Read the model definition and answer for the solid it produces. Units are mm, in the model's axes. A direction names the side the tool comes from. Round coordinates to 2 decimals unless told otherwise and drop trailing zeros. Order: outer loops, then holes, each group sorted by start corner. A loop starts at its lowest first (then second) coordinate and runs counter-clockwise, first axis right, second up. Notation, with made-up numbers: (12.25, -31.5) -> (60.25, -31.5) arc R23 ccw to (60.25, -17.5) -> close; hole circle Ø3 at (86.5, 71). An arc over 180 degrees is marked (long way). Use a Markdown table: item, result. Add a question column.
1. Section A-A, the plane z = -29 is taken. Give the vertices of the cut face in (x, y), then the cut area to 3 significant figures.
2. Given pin 1 (13 mm diameter, centred on x = -25, y = 0, fed in from +Z); pin 2 (3.5 mm diameter, centred on x = -40.5, y = -15.5, fed in from -Z); pin 3 (11.5 mm diameter, centred on y = 7, z = -17, fed in from -X), each flat-ended and moving along its own axis, determine where each tip first touches the part or whether it passes through.
3. Section D-D, the plane x = -10 is taken. Give the vertices of the cut face in (y, z), then the cut area to 3 significant figures.
4. Consider L1, parallel to Y at x = -9.5, z = -2.8; L2, parallel to Y at x = -2.5, z = -28.5; L3, parallel to Y at x = -25, z = -2.2. Determine where each line is inside the solid, lowest interval first. Write a range as [from, to].
5. Section B-B, the plane x = -25 is taken. Give the vertices of the cut face in (y, z), then the cut area to 3 significant figures.
6. For faces 4 (the face through (-50, 0, -2)), 5 (the face through (-2, -0.1, -23.5)), determine the directions among +Z, -Z, +X, -X, +Y, -Y from which every point of the face is accessible in a straight line to the end or side of a thin tool.
7. The mould has two halves that part along Y. Classify faces 1 (the face through (-38, 0, -4)), 2 (the face through (-15.9, 25, -3.8)), 3 (the face through (-2, -2.5, -32)): +Y half, -Y half, draft (parallel to the pull), parting line (faces both ways), or undercut.
8. Section C-C, the plane y = 0 is taken. Give the vertices of the cut face in (x, z), then the cut area to 3 significant figures.
```python
from build123d import *

# Parameters (mm, degrees)
F1_DEPTH = 25
F3_D     = 3.2
F4_D     = 22
F6_DEPTH = 4.001


with BuildPart() as f1:
    # F0 (on Front) → F1 (new body, symmetric)
    with BuildSketch(Plane.XZ):
        Polygon((0, -42), (0, 0), (-50, 0), (-50, -4), (-4, -4), (-4, -42), align=None)
    extrude(amount=F1_DEPTH, both=True)

    # F3 (through all)
    with Locations(Plane.XY):
        with Locations((-9.5, 15.5), (-9.5, -15.5), (-40.5, -15.5), (-40.5, 15.5)):
            Hole(F3_D / 2)

    # F4 (through all)
    with Locations(Plane.XY):
        with Locations((-25, 0)):
            Hole(F4_D / 2)

    # F5 (on face) → F6 (cut, through all)
    with BuildSketch(Plane(origin=(-4, 0, 0), x_dir=(0, -1, 0), z_dir=(-1, 0, 0))):
        with BuildLine():
            ThreePointArc((-17.034974, -22), (-14.534974, -24.5), (-12.034974, -22))
            Line((-12.034974, -22), (-12.034974, -10))
            ThreePointArc((-12.034974, -10), (-14.534974, -7.5), (-17.034974, -10))
            Line((-17.034974, -10), (-17.034974, -22))
        make_face()
        with BuildLine():
            ThreePointArc((-2.5, -38), (0, -40.5), (2.5, -38))
            Line((2.5, -38), (2.5, -26))
            ThreePointArc((2.5, -26), (0, -23.5), (-2.5, -26))
            Line((-2.5, -26), (-2.5, -38))
        make_face()
        with BuildLine():
            ThreePointArc((12.034974, -22), (14.534974, -24.5), (17.034974, -22))
            Line((17.034974, -22), (17.034974, -10))
            ThreePointArc((17.034974, -10), (14.534974, -7.5), (12.034974, -10))
            Line((12.034974, -10), (12.034974, -22))
        make_face()
    extrude(amount=-F6_DEPTH, mode=Mode.SUBTRACT)


solid = f1.part
```
Verdict:
| question | item | result |
|---|---|---|
| 1 | outline | (-4, -25) -> (0, -25) -> (0, -2.5) -> (-4, -2.5) -> close; (-4, 2.5) -> (0, 2.5) -> (0, 25) -> (-4, 25) -> close |
| 1 | area | 180 mm2 |
| 2 | pin 1 | passes through |
| 2 | pin 2 | stops at z = -4 |
| 2 | pin 3 | stops at x = -4 |
| 3 | outline | (-25, -4) -> (-17.02, -4) -> (-17.02, 0) -> (-25, 0) -> close; (-13.98, -4) -> (13.98, -4) -> (13.98, 0) -> (-13.98, 0) -> close; (17.02, -4) -> (25, -4) -> (25, 0) -> (17.02, 0) -> close |
| 3 | area | 176 mm2 |
| 4 | L1 | y = [-25, -17.1], [-13.9, 13.9], [17.1, 25] |
| 4 | L2 | y = [-25, -2.5], [2.5, 25] |
| 4 | L3 | y = [-25, -11], [11, 25] |
| 5 | outline | (-25, -4) -> (-11, -4) -> (-11, 0) -> (-25, 0) -> close; (11, -4) -> (25, -4) -> (25, 0) -> (11, 0) -> close |
| 5 | area | 112 mm2 |
| 6 | face 4 | +Z, -Z, -X, +Y, -Y |
| 6 | face 5 | +X, -X |
| 7 | face 1 | draft |
| 7 | face 2 | +Y half |
| 7 | face 3 | undercut |
| 8 | outline | (-50, -4) -> (-36, -4) -> (-36, 0) -> (-50, 0) -> close; (-14, -4) -> (-4, -4) -> (-4, -23.5) -> (0, -23.5) -> (0, 0) -> (-14, 0) -> close; (-4, -42) -> (0, -42) -> (0, -40.5) -> (-4, -40.5) -> close |
| 8 | area | 196 mm2 |
